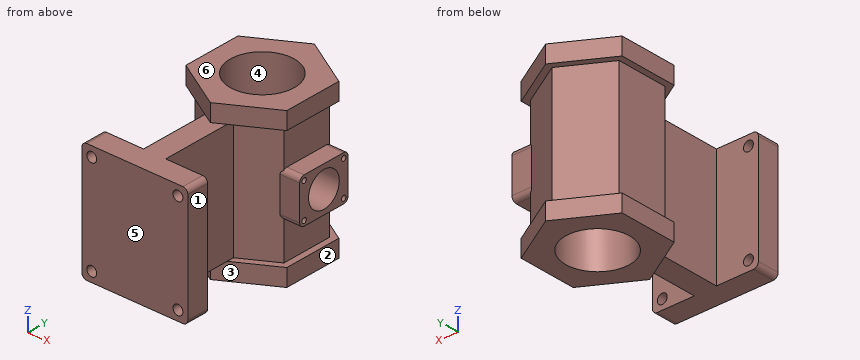
from build123d import *

# Parameters (mm, degrees)
EXTRUDE_1_DEPTH          = 240
EXTRUDE_2_DEPTH          = 35
EXTRUDE_4_DEPTH          = 35
EXTRUDE_5_DEPTH          = 35
EXTRUDE_5_DEPTH_BACK     = 90
SKETCH_5_W               = 90
SKETCH_5_H               = 110
SKETCH_6_R               = 65
CUT_EXTRUDE_1_DEPTH      = 443.521185934
CUT_EXTRUDE_2_REACH      = 464.365
CUT_EXTRUDE_2_END_RADIUS = 65
SKETCH_8_R               = 35
CUT_EXTRUDE_3_REACH      = 509.942
SKETCH_9_R               = 10
SKETCH_10_R              = 5
CUT_EXTRUDE_4_DEPTH      = 30
FILLET_1_R               = 10
FILLET_2_R               = 10


with BuildPart() as part:
    # Эскиз1 → Бобышка-Вытянуть1 (new body)
    with BuildSketch(Plane.XY):
        Polygon((0, 103.923048454), (-90, 51.961524227), (-90, -51.961524227), (-22.5, -90.932667397), (-22.5, -245), (-107.5, -245), (-107.5, -290), (107.5, -290), (107.5, -245), (22.5, -245), (22.5, -90.932667397), (90, -51.961524227), (90, 51.961524227), align=None)
    extrude(amount=EXTRUDE_1_DEPTH)

    # Эскиз2 → Бобышка-Вытянуть2 (add)
    with BuildSketch(Plane.XY.offset(240)):
        Polygon((0, 118.356805184), (-102.5, 59.178402592), (-102.5, -59.178402592), (0, -118.356805184), (102.5, -59.178402592), (102.5, 59.178402592), align=None)
    extrude(amount=EXTRUDE_2_DEPTH)

    # Эскиз4 → Бобышка-Вытянуть4 (add)
    with BuildSketch(Plane(origin=(0, 0, 0), x_dir=(-1, 0, 0), z_dir=(0, 0, -1))):
        Polygon((0, 118.356805184), (-102.5, 59.178402592), (-102.5, -59.178402592), (0, -118.356805184), (102.5, -59.178402592), (102.5, 59.178402592), align=None)
    extrude(amount=EXTRUDE_4_DEPTH)

    # Эскиз5 → Бобышка-Вытянуть5 (add, two sides: drawn at the far end of the back side and taken through both)
    with BuildSketch(Plane(origin=(90, 0, 0), x_dir=(0, 0, -1), z_dir=(1, 0, 0)).offset(-EXTRUDE_5_DEPTH_BACK)):
        with Locations((-120, 0)):
            Rectangle(SKETCH_5_W, SKETCH_5_H)
    extrude(amount=EXTRUDE_5_DEPTH + EXTRUDE_5_DEPTH_BACK)

    # Эскиз6 → Вырез-Вытянуть1 (cut, through all)
    with BuildSketch(Plane.XY.offset(275)):
        Circle(SKETCH_6_R)
    extrude(amount=-CUT_EXTRUDE_1_DEPTH, mode=Mode.SUBTRACT)

    # Вырез-Вытянуть2: up to this cylinder (the profile starts outside it)
    cut_extrude_2_end = Plane(origin=(0, 0, 120), z_dir=(0, 0, 1)) * Cylinder(CUT_EXTRUDE_2_END_RADIUS, 1059.73, mode=Mode.PRIVATE)
    # Эскиз8 → Вырез-Вытянуть2 (cut, up to the surface)
    with BuildSketch(Plane(origin=(125, 0, 0), x_dir=(0, 0, -1), z_dir=(1, 0, 0)), mode=Mode.PRIVATE) as cut_extrude_2_sk1:
        with Locations(Location((-120, 0, 0), (0, 0, 90))):
            Circle(SKETCH_8_R)
    cut_extrude_2_tool1 = extrude(cut_extrude_2_sk1.sketch, amount=-CUT_EXTRUDE_2_REACH, mode=Mode.PRIVATE) - cut_extrude_2_end
    add(cut_extrude_2_tool1.solids().sort_by_distance((125, 0, 120))[0], mode=Mode.SUBTRACT)

    # Эскиз9 → Вырез-Вытянуть3 (cut, up to next)
    with BuildSketch(Plane.XZ.offset(290), mode=Mode.PRIVATE) as cut_extrude_3_sk1:
        with Locations(Location((87.5, 220, 0), (0, 0, 270))):
            Circle(SKETCH_9_R)
    cut_extrude_3_tool1 = extrude(cut_extrude_3_sk1.sketch, amount=-CUT_EXTRUDE_3_REACH, mode=Mode.PRIVATE) & part.part
    # Эскиз9 → Вырез-Вытянуть3 (cut, up to next)
    with BuildSketch(Plane.XZ.offset(290), mode=Mode.PRIVATE) as cut_extrude_3_sk2:
        with Locations(Location((-87.5, 220, 0), (0, 0, 270))):
            Circle(SKETCH_9_R)
    cut_extrude_3_tool2 = extrude(cut_extrude_3_sk2.sketch, amount=-CUT_EXTRUDE_3_REACH, mode=Mode.PRIVATE) & part.part
    # Эскиз9 → Вырез-Вытянуть3 (cut, up to next)
    with BuildSketch(Plane.XZ.offset(290), mode=Mode.PRIVATE) as cut_extrude_3_sk3:
        with Locations(Location((87.5, 20, 0), (0, 0, 270))):
            Circle(SKETCH_9_R)
    cut_extrude_3_tool3 = extrude(cut_extrude_3_sk3.sketch, amount=-CUT_EXTRUDE_3_REACH, mode=Mode.PRIVATE) & part.part
    # Эскиз9 → Вырез-Вытянуть3 (cut, up to next)
    with BuildSketch(Plane.XZ.offset(290), mode=Mode.PRIVATE) as cut_extrude_3_sk4:
        with Locations(Location((-87.5, 20, 0), (0, 0, 270))):
            Circle(SKETCH_9_R)
    cut_extrude_3_tool4 = extrude(cut_extrude_3_sk4.sketch, amount=-CUT_EXTRUDE_3_REACH, mode=Mode.PRIVATE) & part.part
    add(cut_extrude_3_tool1.solids().sort_by_distance((87.5, -290, 220))[0], mode=Mode.SUBTRACT)
    add(cut_extrude_3_tool2.solids().sort_by_distance((-87.5, -290, 220))[0], mode=Mode.SUBTRACT)
    add(cut_extrude_3_tool3.solids().sort_by_distance((87.5, -290, 20))[0], mode=Mode.SUBTRACT)
    add(cut_extrude_3_tool4.solids().sort_by_distance((-87.5, -290, 20))[0], mode=Mode.SUBTRACT)

    # Эскиз10 → Вырез-Вытянуть4 (cut)
    with BuildSketch(Plane(origin=(125, 0, 0), x_dir=(0, 0, -1), z_dir=(1, 0, 0))):
        with Locations(Location((-155, -45, 0), (0, 0, 90))):
            Circle(SKETCH_10_R)
        with Locations(Location((-155, 45, 0), (0, 0, 90))):
            Circle(SKETCH_10_R)
        with Locations(Location((-85, 45, 0), (0, 0, 90))):
            Circle(SKETCH_10_R)
        with Locations(Location((-85, -45, 0), (0, 0, 90))):
            Circle(SKETCH_10_R)
    extrude(amount=-CUT_EXTRUDE_4_DEPTH, mode=Mode.SUBTRACT)

    # Скругление1
    fillet_1_edges = [part.edges().sort_by_distance(p)[0] for p in [
        (104.868602792, -55, 165),
        (104.868602792, -55, 75),
        (104.868602792, 55, 75),
        (104.868602792, 55, 165),
    ]]
    fillet(fillet_1_edges, radius=FILLET_1_R)

    # Скругление2
    fillet_2_edges = [part.edges().sort_by_distance(p)[0] for p in [
        (107.5, -267.5, 0),
        (-107.5, -267.5, 0),
        (-107.5, -267.5, 240),
        (107.5, -267.5, 240),
    ]]
    fillet(fillet_2_edges, radius=FILLET_2_R)


solid = part.part
Work out the finished part from the listing and answer in its coordinate system (mm). Face numbers are marked on the shaded views. A direction names the side the tool comes from. Give positions to 0.01 mm unless a question says otherwise; leave off trailing zeros. Order: outer loops, then holes, each group sorted by start corner. A loop starts at its lowest first (then second) coordinate and runs counter-clockwise, first axis right, second up. Notation, with made-up numbers: M -21,76 L 6,76 A29 ccw 6,115 Z; hole C 69.5,54.25 d3. An arc over 180 degrees is marked long. Return JSON: item names as keys, results as strings.
Q1. Find section D-D, the plane z = 201. Write down the section's boundary in (x, y).
Answer below:
{"outline": "M -107.5,-290 L 107.5,-290 L 107.5,-245 L 22.5,-245 L 22.5,-90.93 L 90,-51.96 L 90,51.96 L 0,103.92 L -90,51.96 L -90,-51.96 L -22.5,-90.93 L -22.5,-245 L -107.5,-245 Z; hole C 0,0 d130"}
Q2. Find section B-B, the plane x = 72. Write down the section's boundary in (y, z), and give its area (3 significant figures).
Answer below:
{"outline": "M -290,0 L -245,0 L -245,240 L -290,240 Z; M -76.79,-35 L 76.79,-35 L 76.79,0 L 62.35,0 L 62.35,240 L 76.79,240 L 76.79,275 L -76.79,275 L -76.79,240 L -62.35,240 L -62.35,0 L -76.79,0 Z; hole C 0,120 d70", "area": "47,600 mm^2"}
Q3. Each of these flat-tipped pins is pushed along its axis until it touches: pin 1 (12 mm diameter, centred on x = 76.5, z = 160, fed in from +Y); pin 2 (8 mm diameter, centred on y = -45, z = 155, fed in from +X); pin 3 (17.5 mm diameter, centred on y = 7, z = 251.5, fed in from +X). Where does it stop, or does it pass through?
Answer below:
{"pin 1": "stops at y = 63.22", "pin 2": "stops at x = 95", "pin 3": "stops at x = 102.5"}
Q4. Find section C-C, the plane y = 0. Write down the section's boundary in (x, z), and give its area (3 significant figures).
Answer below:
{"outline": "M -102.5,-35 L -65,-35 L -65,275 L -102.5,275 L -102.5,240 L -90,240 L -90,0 L -102.5,0 Z; M 65,-35 L 102.5,-35 L 102.5,0 L 90,0 L 90,75 L 125,75 L 125,85 L 65,85 Z; M 65,155 L 125,155 L 125,165 L 90,165 L 90,240 L 102.5,240 L 102.5,275 L 65,275 Z", "area": "16,200 mm^2"}
Q5. Find section A-A, the plane z = 20. Write down the section's boundary in (x, y).
Answer below:
{"outline": "M -107.5,-290 L -97.5,-290 L -97.5,-245 L -107.5,-245 Z; M -90,-51.96 L -22.5,-90.93 L -22.5,-245 L -77.5,-245 L -77.5,-290 L 77.5,-290 L 77.5,-245 L 22.5,-245 L 22.5,-90.93 L 90,-51.96 L 90,51.96 L 0,103.92 L -90,51.96 Z; M 97.5,-290 L 107.5,-290 L 107.5,-245 L 97.5,-245 Z; hole C 0,0 d130"}
Q6. Which of the six approach directions +Z, -Z, +X, -X, +Y, -Y give full straight-line access (tool end or side, diameter ignored) to the marked faces 1, 2 and 3?
Answer below:
{"face 1": "+Z, -Z, +X, -Y", "face 2": "-Z, +X, +Y, -Y", "face 3": "-Z, +X, -Y"}
Q7. The mould has two halves that part along Y. Classify the marked faces 4, 5 and 6: pulls with the +Y half, pulls with the -Y half, needs draft (parallel to the pull), parting line crosses it, or undercut.
Answer below:
{"face 4": "undercut", "face 5": "pulls with the -Y half", "face 6": "needs draft"}
Q8. Find the intervals of material crossed by line 1 along Y through (x, z) = (107, 120); line 2 along X through (y, z) = (-278.5, 220); line 3 along X through (y, z) = (-253, 228), in increasing order. Write a range as [from, to].
Answer below:
{"line 1": "y = [-290, -245], [-55, -35], [35, 55]", "line 2": "x = [-107.5, -97.5], [-77.5, 77.5], [97.5, 107.5]", "line 3": "x = [-107.5, -93.5], [-81.5, 81.5], [93.5, 107.5]"}
